Source: CAD feature listing. Evaluate the final solid. Frame: model axes, mm. Face numbers are marked on the shaded views. A direction names the side the tool comes from. Give positions to 0.01 mm unless a question says otherwise; leave off trailing zeros. Write each loop counter-clockwise with the first axis right and the second up, starting at its lowest first coordinate (ties: lowest second). Pieces come first, ordered by that corner, then holes. Notation, with made-up numbers: (-16.75, 24.25) -> (39.25, 24.25) arc R21 ccw to (39.25, 30.25) -> close; hole circle Ø5 at (1, 68). An arc over 180 degrees is marked (long way). Write item = value, one per line.
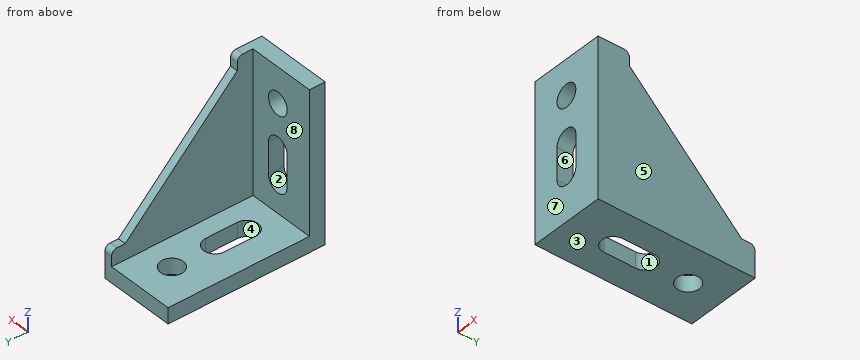
from build123d import *

# Parameters (mm, degrees)
SKETCH_1_W          = 28
SKETCH_1_H          = 58
EXTRUDE_1_DEPTH     = 5.8
SKETCH_2_W          = 28
SKETCH_2_H          = 5.8
EXTRUDE_2_DEPTH     = 58
EXTRUDE_3_DEPTH     = 3
FILLET_1_R          = 2
SKETCH_4_R          = 4.15
CUT_EXTRUDE_1_DEPTH = 80.276982788


with BuildPart() as part:
    # 草图1 → 凸台-拉伸1 (new body)
    with BuildSketch(Plane.XY):
        Rectangle(SKETCH_1_W, SKETCH_1_H)
    extrude(amount=EXTRUDE_1_DEPTH)

    # 草图2 → 凸台-拉伸2 (add)
    with BuildSketch(Plane(origin=(0, 0, 0), x_dir=(-1, 0, 0), z_dir=(0, 0, -1))):
        with Locations((0, -26.1)):
            Rectangle(SKETCH_2_W, SKETCH_2_H)
    extrude(amount=-EXTRUDE_2_DEPTH)

    # 草图3 → 凸台-拉伸3 (add)
    with BuildSketch(Plane(origin=(14, 0, 0), x_dir=(0, 0, -1), z_dir=(1, 0, 0))):
        Polygon((-5.8, 29), (-11.6, 29), (-11.6, 24), (-53, -17.4), (-58, -17.4), (-58, -23.2), (-5.8, -23.2), align=None)
    extrude(amount=-EXTRUDE_3_DEPTH)

    # 圆角1
    fillet_1_edges = [part.edges().sort_by_distance(p)[0] for p in [
        (12.5, -17.4, 58),
        (12.5, 29, 11.6),
    ]]
    fillet(fillet_1_edges, radius=FILLET_1_R)

    # 草图4 → 切除-拉伸1 (cut, through all)
    with BuildSketch(Plane(origin=(0, -23.2, 0), x_dir=(1, 0, 0), z_dir=(0, 1, 0))):
        with Locations(Location((0, -44.929446332, 0), (0, 0, 180))):
            Circle(SKETCH_4_R)
        with BuildLine():
            Line((4.15, -17.270397055), (4.15, -28.970397055))
            ThreePointArc((4.15, -28.970397055), (0, -33.120397055), (-4.15, -28.970397055))
            Line((-4.15, -28.970397055), (-4.15, -17.270397055))
            ThreePointArc((-4.15, -17.270397055), (0, -13.120397055), (4.15, -17.270397055))
        make_face()
    cut_extrude_1 = extrude(amount=-CUT_EXTRUDE_1_DEPTH, mode=Mode.SUBTRACT)

    # 镜向1: 切除-拉伸1 across plane
    add(cut_extrude_1.mirror(Plane(origin=(0, -14.5, 14.5), x_dir=(0, 0.7071067811865469, 0.7071067811865482), z_dir=(0, -0.7071067811865483, 0.7071067811865468))), mode=Mode.SUBTRACT)


solid = part.part
(1) First-contact query: pin 1 (12 mm diameter, centred on x = -6, z = 19.5, fed in from +Y); pin 2 (0.9 mm diameter, centred on x = 12, y = 26, fed in from +Z); pin 3 (4 mm diameter, centred on x = 1.5, y = 16, fed in from +Z); pin 4 (12.5 mm diameter, centred on x = -1.5, y = -2.5, fed in from +Z). Flat tips, straight axial feed; report the tip coordinate or a pass-through.
Values follow:
pin_1 = -23.2
pin_2 = 11.6
pin_3 = through
pin_4 = 5.8
(2) Material intervals for line 1 (Y direction, x = 0, z = 4.35); line 2 (Z direction, x = 0, y = -26.8); line 3 (Z direction, x = 7.25, y = 14), sorted ascending.
Values follow:
line_1 = -29 to -15.88, 4.12 to 11.78, 20.08 to 29
line_2 = 0 to 13.12, 33.12 to 40.78, 49.08 to 58
line_3 = 0 to 5.8
(3) Section query A-A (x = 0). Return loops of the section in (y, z), plus the area to 3 significant figures.
Values follow:
outline = (-29, 0) -> (-15.88, 0) -> (-15.88, 5.8) -> (-23.2, 5.8) -> (-23.2, 13.12) -> (-29, 13.12) -> close; (-29, 33.12) -> (-23.2, 33.12) -> (-23.2, 40.78) -> (-29, 40.78) -> close; (-29, 49.08) -> (-23.2, 49.08) -> (-23.2, 58) -> (-29, 58) -> close; (4.12, 0) -> (11.78, 0) -> (11.78, 5.8) -> (4.12, 5.8) -> close; (20.08, 0) -> (29, 0) -> (29, 5.8) -> (20.08, 5.8) -> close
area = 311 mm2
(4) Section query C-C (z = 47). Return loops of the section in (x, y).
Values follow:
outline = (-14, -29) -> (-3.6, -29) -> (-3.6, -23.2) -> (-14, -23.2) -> close; (3.6, -29) -> (14, -29) -> (14, -11.4) -> (11, -11.4) -> (11, -23.2) -> (3.6, -23.2) -> close
(5) Section query D-D (z = 34). Return loops of the section in (x, y), plus the area to 3 significant figures.
Values follow:
outline = (-14, -29) -> (14, -29) -> (14, 1.6) -> (11, 1.6) -> (11, -23.2) -> (-14, -23.2) -> close
area = 237 mm2
(6) Pull-direction query (Z, two-part tool) for the marked faces 1, 2 and 3; classes: pulls with the +Z half, pulls with the -Z half, needs draft (parallel to the pull), parting line crosses it, or undercut.
Values follow:
face_1 = needs draft
face_2 = undercut
face_3 = pulls with the -Z half
(7) Access query for the marked faces 4, 5, 6, 7 and 8. Directions: +Z, -Z, +X, -X, +Y, -Y. A direction counts if a zero-diameter tool reaches every point of the face in a straight line with its end or side. Return the directions, or none.
Values follow:
face_4 = +Z, -Z
face_5 = +Z, -Z, +X, +Y, -Y
face_6 = +Y, -Y
face_7 = +Z, -Z, +X, -X, -Y
face_8 = +Z, -X, +Y
(8) Section query B-B (y = -9.5). Return loops of the section in (x, z).
Values follow:
outline = (-14, 0) -> (-4.15, 0) -> (-4.15, 5.8) -> (-14, 5.8) -> close; (4.15, 0) -> (14, 0) -> (14, 45.1) -> (11, 45.1) -> (11, 5.8) -> (4.15, 5.8) -> close
